Part model, mm, in its own coordinate system. A direction names the side the tool comes from. Round coordinates to 2 decimals unless told otherwise and drop trailing zeros. Loops run counter-clockwise (first coordinate to the right, second up) from the corner with the lowest first, then second, coordinate; pieces in that order, holes last. Notation, with made-up numbers: M 55,49 L 59,49 A22 cw 59,71 Z; hole C -1,21.25 d11. An arc over 180 degrees is marked long. Write each question's results on one line, items separated by ' | '.
Autodesk Inventor part; units mm, degrees
ref_plane "YZ Plane" through (0, 0, 0) normal (1, 0, 0) x (0, 1, 0)
ref_plane "XZ Plane" through (0, 0, 0) normal (0, 1, 0) x (-1, 0, 0)
ref_plane "XY Plane" through (0, 0, 0) normal (0, 0, 1) x (1, 0, 0)
sketch "Sketch1" plane through (0, 0, 0) normal (0, 1, 0) x (-1, 0, 0)
  circle A0 centre (0, 0) radius 12.7
  circle A1 centre (0, 0) radius 3.302
  dimension "d0" = 25.4
  dimension "d1" = 6.604
extrude "Extrusion1" add sketch "Sketch1" along normal blind 19.558
sketch "Sketch2" plane through (0, 19.558, 0) normal (0, 1, 0) x (1, 0, 0)
  line L0 (0, 0) -> (0, -5.004)
  line L1 (0, -5.004) -> (0, 0)
  line L2 (0, 0) -> (0, 5.004)
  circle A0 centre (0, -5.004) radius 1.0125
  circle A1 centre (0, 5.004) radius 1.0125
  dimension "d4" = 5.004
  dimension "d5" = 5.004
  dimension "d6" = 2.025
  dimension "d7" = 2.025
extrude "Extrusion2" cut sketch "Sketch2" against normal blind 4.445
sketch "Sketch3" plane through (0, 0, 0) normal (0, -1, 0) x (1, 0, 0)
  line L0 (0, 0) -> (0, 5.004)
  line L1 (0, 5.004) -> (0, -5.08)
  circle A0 centre (0, 5.004) radius 1.0125
  line L2 (0, 0) -> (0, -5.004)
  circle A1 centre (0, -5.08) radius 1.0125
  dimension "d10" = 5.004
  dimension "d15" = 2.025
  dimension "d16" = 5.004
  dimension "d17" = 2.025
extrude "Extrusion3" cut sketch "Sketch3" against normal blind 4.445
properties part number "PolarisPost_HeightAdjustment_0p5in_Machined"
Item 1: Two-plate mould, pull along X, no slides. Class faces 4 (the cylindrical face through (2.75, 9.64, 12.4)), 5 (the flat face through (-3, 19.558, -3)), 6 (the flat face through (0, 15.113, 5)): +X half, -X half, draft (parallel to the pull), parting line (faces both ways), or undercut.
Filled sheet:
face 4: parting line | face 5: draft | face 6: undercut
Item 2: Drop flat-ended pins along their axis: P1, Ø2.5, axis at x = 0, z = -5.004, coming from the +Y side; P2, Ø1, axis at y = 15, z = 7, coming from the +X side; P3, Ø1.6, axis at x = 0, z = 5, coming from the +Y side; P4, Ø4, axis at x = 0, z = 0, coming from the +Y side. Give the stop position or say it passes through.
Filled sheet:
P1: y = 19.56 | P2: x = 10.91 | P3: y = 15.11 | P4: through
Item 3: Wall check: L1, parallel to Z at x = 0, y = 2.45; L2, parallel to X at y = 17.75, z = -1.75; L3, parallel to Z at x = -3, y = 8.25. Give the ranges that are in metal, low to high.
Filled sheet:
L1: -12.7 to -6.09, -4.07 to -3.3, 3.3 to 3.99, 6.02 to 12.7 | L2: -12.58 to -2.8, 2.8 to 12.58 | L3: -12.34 to -1.38, 1.38 to 12.34
Item 4: Band-saw the part on A-A on x = 0. Give the cut face in (y, z) (1 decimal), and give its area (3 significant figures).
Filled sheet:
outline: M 0,-12.7 L 19.6,-12.7 L 19.6,-6 L 15.1,-6 L 15.1,-4 L 19.6,-4 L 19.6,-3.3 L 0,-3.3 L 0,-4.1 L 4.4,-4.1 L 4.4,-6.1 L 0,-6.1 Z; M 0,3.3 L 19.6,3.3 L 19.6,4 L 15.1,4 L 15.1,6 L 19.6,6 L 19.6,12.7 L 0,12.7 L 0,6 L 4.4,6 L 4.4,4 L 0,4 Z | area: 332 mm^2
Item 5: Band-saw the part on B-B on z = 0. Give the cut face in (x, y), and give its area (3 significant figures).
Filled sheet:
outline: M -12.7,0 L -3.3,0 L -3.3,19.56 L -12.7,19.56 Z; M 3.3,0 L 12.7,0 L 12.7,19.56 L 3.3,19.56 Z | area: 368 mm^2
Item 6: Band-saw the part on C-C on y = 11.25. Give the cut face in (x, z).
Filled sheet:
outline: C 0,0 d25.4; hole C 0,0 d6.6
Item 7: Band-saw the part on D-D on x = 7.5. Give the cut face in (y, z).
Filled sheet:
outline: M 0,-10.25 L 19.56,-10.25 L 19.56,10.25 L 0,10.25 Z
Item 8: Which spindle directions (+Z, -Z, +X, -X, +Y, -Y) get a long thin tool onto all of the face, cutting with end or side? Do faces 1 (the cylindrical face through (-0.13, 17.37, -6.01)), 2 (the cylindrical face through (-0.13, 2.19, 6.01)), 3 (the flat face through (-3, 0, -3)). Say none if no direction does.
Filled sheet:
face 1: +Y | face 2: -Y | face 3: +Z, -Z, +X, -X, -Y
